from build123d import *
from build123d import SkipClean  # not in build123d's __all__

# Parameters (mm, degrees)
F0_R      = 7
F1_DEPTH  = 75
F2_R      = 1
F3_DEPTH  = 150.001
F4_R      = 5.5
F4_R_2    = 1
F5_DEPTH  = 8
F6_W      = 0.5
F6_H      = 0.5
F13_R     = 4
F14_DEPTH = 40
F16_R     = 1
F17_DEPTH = 40
F18_R     = 4
F19_DEPTH = 40
F20_R     = 1
F21_DEPTH = 33


with BuildPart() as f1:
    # F0 (on Right) → F1 (new body, symmetric)
    with BuildSketch(Plane.YZ):
        Circle(F0_R)
    extrude(amount=F1_DEPTH, both=True)

    # F2 (on face) → F3 (cut, through all)
    with BuildSketch(Plane(origin=(-75, 0, 0), x_dir=(0, -1, 0), z_dir=(-1, 0, 0))):
        Circle(F2_R)
    extrude(amount=-F3_DEPTH, mode=Mode.SUBTRACT)

    # F4 (on face) → F5 (cut)
    with BuildSketch(Plane(origin=(-75, 0, 0), x_dir=(0, -1, 0), z_dir=(-1, 0, 0))):
        Circle(F4_R)
        Circle(F4_R_2, mode=Mode.SUBTRACT)
    extrude(amount=-F5_DEPTH, mode=Mode.SUBTRACT)

    # F6 (on Top) → F7 (revolve, cut)
    with BuildSketch(Plane.XY):
        with Locations((-66.75, 1.75)):
            Rectangle(F6_W, F6_H)
    revolve(axis=Axis((-60.2624397725, 0, 0), (1, 0, 0)), mode=Mode.SUBTRACT)

    # F13 (on face) → F14 (join)
    with BuildSketch(Plane(origin=(33.8824944498, 21.5843530986, -15.7996666393), x_dir=(-0.4531538935, 0.8660254038, 0.2113091309), z_dir=(0.7848855672, 0.5, -0.3659981508))):
        with Locations((-24.9234641435, 23.2440043957)):
            Circle(F13_R)
    extrude(amount=F14_DEPTH)

    # F16 (on face) → F17 (cut)
    with BuildSketch(Plane(origin=(65.2779171386, 41.5843530986, -30.4395926702), x_dir=(-0.4531538935, 0.8660254038, 0.2113091309), z_dir=(0.7848855672, 0.5, -0.3659981508))):
        with Locations((-24.9234641435, 23.2440043957)):
            Circle(F16_R)
    extrude(amount=-F17_DEPTH, mode=Mode.SUBTRACT)

    # F18 (on face) → F19 (join)
    with BuildSketch(Plane(origin=(33.8824944498, -21.5843530986, -15.7996666393), x_dir=(-0.4531538935, -0.8660254038, 0.2113091309), z_dir=(-0.7848855672, 0.5, 0.3659981508))):
        with Locations((-24.9234641435, 23.2440043957)):
            Circle(F18_R)
    with SkipClean():  # cleaning this boolean's faces spoils the solid; the shape is the same uncleaned
        extrude(amount=-F19_DEPTH)

    # F20 (on face) → F21 (cut)
    with BuildSketch(Plane(origin=(65.2779171386, -41.5843530986, -30.4395926702), x_dir=(0.4531538935, 0.8660254038, -0.2113091309), z_dir=(0.7848855672, -0.5, -0.3659981508))):
        with Locations((24.9234641435, 23.2440043957)):
            Circle(F20_R)
    with SkipClean():  # cleaning this boolean's faces spoils the solid; the shape is the same uncleaned
        extrude(amount=-F21_DEPTH, mode=Mode.SUBTRACT)


solid = f1.part
Verification items for the finished model (mm, model axes). A direction names the side the tool comes from. Coordinates: 2 decimals unless noted, no trailing zeros. Loops run counter-clockwise (first coordinate to the right, second up) from the corner with the lowest first, then second, coordinate; pieces in that order, holes last. Notation, with made-up numbers: (28, 76.25) -> (57, 76.25) arc R16 cw to (57, 90.25) -> close; hole circle Ø8 at (47.5, 71.5). An arc over 180 degrees is marked (long way). Write each question's results on one line, items separated by ' | '.
Item 1: Section check A-A, the plane x = -26.5. Enter the section's corners in (y, z).
Found:
outline: circle Ø14 at (0, 0); hole circle Ø2 at (0, 0)
Item 2: Section check B-B, the plane x = 73.5. Count the separate pieces of the cut face and the enclosed holes in it, plus the area to 3 significant figures.
Found:
separate pieces: 3 | enclosed holes: 3 | area: 271 mm2
Item 3: Material ranges on L1, parallel to Z at x = -66, y = 0; L2, parallel to Z at x = -72, y = 0; L3, parallel to X at y = 2.5, z = 3.25, recorded low to high.
Found:
L1: z = -7 to -1, 1 to 7 | L2: z = -7 to -5.5, 5.5 to 7 | L3: x = -67 to 75
Item 4: Mould release check, pull along Y, two halves, no side actions. Record for faces 3 (the face through (85.666, 20.721, -15.219)), 4 (the face through (-75, -4, -4)), 5 (the face through (70.62, -13.04, -11.2)): +Y half, -Y half, draft (parallel to the pull), parting line (faces both ways), or undercut.
Found:
face 3: +Y half | face 4: draft | face 5: undercut
Item 5: Gauge pin test, flat ends, axial feed: pin 1 (6 mm diameter, centred on x = -3, z = -4, fed in from +Y); pin 2 (10 mm diameter, centred on x = -24, z = -3, fed in from +Y); pin 3 (0.9 mm diameter, centred on y = 0, z = 0, fed in from -X); pin 4 (5 mm diameter, centred on x = -48, y = -10.5, fed in from -Z). Record the tip position at first contact, or that the pin passes through.
Found:
pin 1: stops at y = 6.93 | pin 2: stops at y = 7 | pin 3: stops at x = 54.64 | pin 4: passes through
Item 6: Tool access check on faces 1 (the face through (-67, 0.1, -2.4)), 2 (the face through (72, 12, -8)). Record the directions out of +Z, -Z, +X, -X, +Y, -Y that give a thin tool (end or side, any length) a straight path to the whole face; none if there is none.
Found:
face 1: -X | face 2: none
